Check sheet for the modelled part. Datum: model origin and axes. Units: mm. A direction names the side the tool comes from. Coordinates: 2 decimals unless noted, no trailing zeros. Write each loop counter-clockwise with the first axis right and the second up, starting at its lowest first coordinate (ties: lowest second). Pieces come first, ordered by that corner, then holes. Notation, with made-up numbers: (85.25, 86) - (110.25, 86) arc R12 ccw to (110.25, 106) - close; hole circle Ø3 at (3, 7). An arc over 180 degrees is marked (long way). Use one line per item in the form item = value. Start each with the question number.
1. Draft check along Y on faces 1 (the face through (-22, 43.812, 19)), 2 (the face through (0, -12, 3.302)), 3 (the face through (12.827, -18, 2)). Enter one of: +Y half, -Y half, draft (parallel to the pull), parting line (faces both ways), or undercut.
2. Cross-section at D-D on x = 15. Record the boundary of the cut face in (y, z), then the cut area to 3 significant figures.
3. Scan lines: line 1 along X through (y, z) = (31.5, 23); line 2 along Y through (x, z) = (-26.5, 2); line 3 along Z through (x, y) = (0.5, -8.5). Record each from-to range of solid material in increasing order.
4. Cross-section at C-C on z = 10.5. Record the boundary of the cut face in (x, y).
5. Tool access check on faces 4 (the face through (1.67, -42.82, 18.78)), 5 (the face through (-12.827, -18, 2)), 6 (the face through (0, 4.188, 19)), 7 (the face through (12.827, -18, 36)). Record the directions out of +Z, -Z, +X, -X, +Y, -Y that give a thin tool (end or side, any length) a straight path to the whole face; none if there is none.
6. Cross-section at A-A on y = 31.5. Record the boundary of the cut face in (x, z), then the cut area to 3 significant figures.
7. Go/stop test with flat-tipped pins: pin 1 Ø5 at (x, y) = (-26.5, -7.5) entering from +Z; pin 2 Ø11 at (x, z) = (22, 11.5) entering from -Y; pin 3 Ø6 at (x, z) = (-2, 7.5) entering from +Y; pin 4 Ø1 at (y, z) = (-18, 36) entering from +X. Record where each tip stops, or that it passes through.
8. Cross-section at B-B on x = 0. Record the boundary of the cut face in (y, z).
```python
from build123d import *

# Parameters (mm, degrees)
SKETCH1_R            = 12.827
BOSS_EXTRUDE1_DEPTH  = 38.1
SKETCH2_W            = 25.654
SKETCH2_H            = 25.4
BOSS_EXTRUDE2_DEPTH  = 3.302
SKETCH8_W            = 63.5
SKETCH8_H            = 38.1
BOSS_EXTRUDE6_DEPTH  = 8.89
SKETCH10_W           = 38.1
SKETCH10_H           = 46.99
BOSS_EXTRUDE7_DEPTH  = 3.048
SKETCH11_W           = 38.1
SKETCH11_H           = 46.99
BOSS_EXTRUDE8_DEPTH  = 3.048
SKETCH13_W           = 25.4
SKETCH13_H           = 38.1
BOSS_EXTRUDE9_DEPTH  = 1.524
SKETCH14_W           = 25.4
SKETCH14_H           = 38.1
BOSS_EXTRUDE10_DEPTH = 1.524
SKETCH16_W           = 25.654
SKETCH16_H           = 25.4
BOSS_EXTRUDE12_DEPTH = 3.302


with BuildPart() as part:
    # Sketch1 → Boss-Extrude1 (new body)
    with BuildSketch(Plane.XY):
        with Locations(Location((0, -30.101764051, 0), (0, 0, 180))):
            Circle(SKETCH1_R)
    extrude(amount=BOSS_EXTRUDE1_DEPTH)

    # Sketch2 → Boss-Extrude2 (add)
    with BuildSketch(Plane.XY):
        with Locations((0, -17.401764051)):
            Rectangle(SKETCH2_W, SKETCH2_H)
    extrude(amount=BOSS_EXTRUDE2_DEPTH)

    # Sketch8 → Boss-Extrude6 (add)
    with BuildSketch(Plane(origin=(0, -4.701764051, 0), x_dir=(1, 0, 0), z_dir=(0, 1, 0))):
        with Locations((0, -19.05)):
            Rectangle(SKETCH8_W, SKETCH8_H)
    extrude(amount=BOSS_EXTRUDE6_DEPTH)

    # Sketch10 → Boss-Extrude7 (add)
    with BuildSketch(Plane(origin=(31.75, 0, 0), x_dir=(0, 0, -1), z_dir=(1, 0, 0))):
        with Locations((-19.05, 18.793235949)):
            Rectangle(SKETCH10_W, SKETCH10_H)
    extrude(amount=BOSS_EXTRUDE7_DEPTH)

    # Sketch11 → Boss-Extrude8 (add)
    with BuildSketch(Plane.ZY.offset(31.75)):
        with Locations((19.05, 18.793235949)):
            Rectangle(SKETCH11_W, SKETCH11_H)
    extrude(amount=BOSS_EXTRUDE8_DEPTH)

    # Sketch13 → Boss-Extrude9 (add)
    with BuildSketch(Plane(origin=(0, 42.288235949, 0), x_dir=(1, 0, 0), z_dir=(0, 1, 0))):
        with Locations((22.098, -19.05)):
            Rectangle(SKETCH13_W, SKETCH13_H)
    extrude(amount=BOSS_EXTRUDE9_DEPTH)

    # Sketch14 → Boss-Extrude10 (add)
    with BuildSketch(Plane(origin=(0, 42.288235949, 0), x_dir=(1, 0, 0), z_dir=(0, 1, 0))):
        with Locations((-22.098, -19.05)):
            Rectangle(SKETCH14_W, SKETCH14_H)
    extrude(amount=BOSS_EXTRUDE10_DEPTH)

    # Sketch16 → Boss-Extrude12 (add)
    with BuildSketch(Plane.XY.offset(38.1)):
        with Locations((0, -17.401764051)):
            Rectangle(SKETCH16_W, SKETCH16_H)
    extrude(amount=-BOSS_EXTRUDE12_DEPTH)


solid = part.part
```
Final values:
q1.face_1 = +Y half
q1.face_2 = undercut
q1.face_3 = draft
q2.outline = (-4.7, 0) - (4.19, 0) - (4.19, 38.1) - (-4.7, 38.1) - close; (42.29, 0) - (43.81, 0) - (43.81, 38.1) - (42.29, 38.1) - close
q2.area = 397 mm²
q3.line_1 = -34.8 to -31.75, 31.75 to 34.8
q3.line_2 = -4.7 to 4.19, 42.29 to 43.81
q3.line_3 = 0 to 3.3, 34.8 to 38.1
q4.outline = (-34.8, -4.7) - (34.8, -4.7) - (34.8, 43.81) - (9.4, 43.81) - (9.4, 42.29) - (31.75, 42.29) - (31.75, 4.19) - (-31.75, 4.19) - (-31.75, 42.29) - (-9.4, 42.29) - (-9.4, 43.81) - (-34.8, 43.81) - close; circle Ø25.65 at (0, -30.1)
q5.face_4 = none
q5.face_5 = +Z, -Z, -X, -Y
q5.face_6 = +Z, -Z
q5.face_7 = +Z, -Z, +X, -Y
q6.outline = (-34.8, 0) - (-31.75, 0) - (-31.75, 38.1) - (-34.8, 38.1) - close; (31.75, 0) - (34.8, 0) - (34.8, 38.1) - (31.75, 38.1) - close
q6.area = 232 mm²
q7.pin_1 = through
q7.pin_2 = -4.7
q7.pin_3 = 4.19
q7.pin_4 = 12.83
q8.outline = (-42.93, 0) - (4.19, 0) - (4.19, 38.1) - (-42.93, 38.1) - close; hole (-17.27, 3.3) - (-4.7, 3.3) - (-4.7, 34.8) - (-17.27, 34.8) - close
